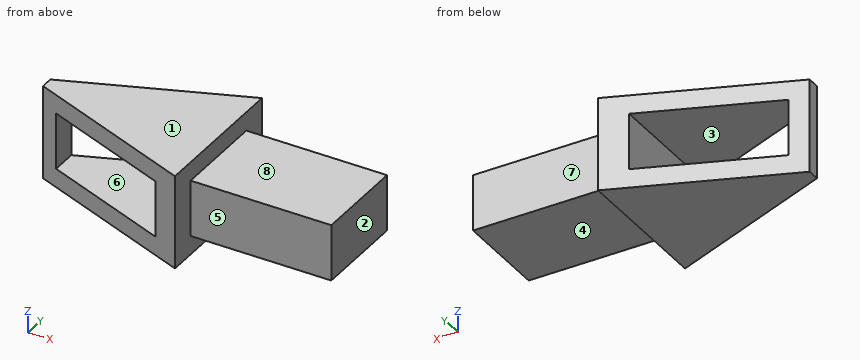
```python
from build123d import *

# Parameters (mm, degrees)
F1_DEPTH = 25.4
F2_W     = 70.138792
F2_H     = 30.48
F3_DEPTH = 63.5
F5_DEPTH = 25.4
F6_W     = 76.2
F6_H     = 25.4
F7_DEPTH = 15.24


with BuildPart() as f1:
    # F0 (on Top) → F1 (new body, symmetric)
    with BuildSketch(Plane.XY):
        Polygon((0, -36.525619), (0, 39.674381), (-101.6, 0), align=None)
    extrude(amount=F1_DEPTH, both=True)

    # F2 (on Front) → F3 (cut, symmetric)
    with BuildSketch(Plane.XZ):
        with Locations((-48.750604, 0)):
            Rectangle(F2_W, F2_H)
    extrude(amount=F3_DEPTH, both=True, mode=Mode.SUBTRACT)

    # F4 (on Top) → F5 (cut, symmetric)
    with BuildSketch(Plane.XY):
        Polygon((-93.059749, 3.334933), (-101.6, 0), (-93.059749, -3.070255), align=None)
    extrude(amount=F5_DEPTH, both=True, mode=Mode.SUBTRACT)

    # F6 (on Top) → F7 (join, symmetric)
    with BuildSketch(Plane.XY):
        with Locations((38.1, 12.7)):
            Rectangle(F6_W, F6_H)
    extrude(amount=F7_DEPTH, both=True)

    # F8: F1 across plane


with BuildPart() as f1_1:
    add(f1.part)
    add(f1.part.mirror(Plane.XZ))


solid = f1_1.part
```
Input: part model. Units: mm. Frame: model coordinates. Face numbers are marked on the shaded views. A direction names the side the tool comes from. Coordinates: 2 decimals unless noted, no trailing zeros. Loops run counter-clockwise (first coordinate to the right, second up) from the corner with the lowest first, then second, coordinate; pieces in that order, holes last. Notation, with made-up numbers: (13.25, 79.5) - (28.25, 79.5) arc R27 cw to (28.25, 112.5) - close; hole circle Ø8 at (83.5, -37). An arc over 180 degrees is marked (long way). Answer in a Markdown table with one row per item.
(1) Material intervals for L1, parallel to Z at x = -43, y = -16; L2, parallel to X at y = 2.5, z = -3; L3, parallel to Z at x = 67, y = -20.5, sorted ascending. Write a range as from..to.
Model answer:
| item | result |
|---|---|
| L1 | z = -25.4..-15.24, 15.24..25.4 |
| L2 | x = -93.06..-83.82, -13.68..76.2 |
| L3 | z = -15.24..15.24 |
(2) Cut plane B-B on z = -13. Output: boundary loops of the cut face in (x, y), plus the area to 3 significant figures.
Model answer:
| item | result |
|---|---|
| outline | (-93.06, -3.33) - (-83.82, -6.94) - (-83.82, 6.94) - (-93.06, 3.33) - close; (-13.68, -34.33) - (0, -39.67) - (0, -25.4) - (76.2, -25.4) - (76.2, 25.4) - (0, 25.4) - (0, 39.67) - (-13.68, 34.33) - close |
| area | 4,980 mm² |
(3) Cut plane D-D on y = 31.5. Output: boundary loops of the cut face in (x, z).
Model answer:
| item | result |
|---|---|
| outline | (-20.93, -25.4) - (0, -25.4) - (0, 25.4) - (-20.93, 25.4) - (-20.93, 15.24) - (-13.68, 15.24) - (-13.68, -15.24) - (-20.93, -15.24) - close |
(4) Cut plane C-C on x = -38. Output: boundary loops of the cut face in (y, z), plus the area to 3 significant figures.
Model answer:
| item | result |
|---|---|
| outline | (-24.84, -25.4) - (24.84, -25.4) - (24.84, -15.24) - (-24.84, -15.24) - close; (-24.84, 15.24) - (24.84, 15.24) - (24.84, 25.4) - (-24.84, 25.4) - close |
| area | 1,010 mm² |
(5) Set-up query: the marked faces 5, 6, 7 and 8. Return all of +Z, -Z, +X, -X, +Y, -Y with unobstructed straight access to the full face (end or side cutting, diameter ignored); none if empty.
Model answer:
| item | result |
|---|---|
| face 5 | +Z, -Z, +X, -Y |
| face 6 | +Y, -Y |
| face 7 | +Z, -Z, +X, +Y |
| face 8 | +Z, +X, +Y, -Y |
(6) Cut plane A-A on y = -1.5. Output: boundary loops of the cut face in (x, z), plus the area to 3 significant figures.
Model answer:
| item | result |
|---|---|
| outline | (-93.06, -25.4) - (0, -25.4) - (0, -15.24) - (76.2, -15.24) - (76.2, 15.24) - (0, 15.24) - (0, 25.4) - (-93.06, 25.4) - close; hole (-83.82, -15.24) - (-13.68, -15.24) - (-13.68, 15.24) - (-83.82, 15.24) - close |
| area | 4,910 mm² |
(7) Pin query (flat end, axial travel): P1, Ø5, axis at x = 42.5, y = -16, coming from the +Z side; P2, Ø15, axis at x = 47, z = -0.5, coming from the +Y side; P3, Ø9, axis at y = 16, z = -2, coming from the -X side. Return the tip coordinate at first contact, or that it passes through.
Model answer:
| item | result |
|---|---|
| P1 | stops at z = 15.24 |
| P2 | stops at y = 25.4 |
| P3 | stops at x = -13.68 |
(8) Mould query, pull axis Z, two halves, no side actions, for the marked faces 1, 2, 3 and 4. Classes: pulls with the +Z half, pulls with the -Z half, needs draft (parallel to the pull), parting line crosses it, or undercut.
Model answer:
| item | result |
|---|---|
| face 1 | pulls with the +Z half |
| face 2 | needs draft |
| face 3 | undercut |
| face 4 | pulls with the -Z half |
